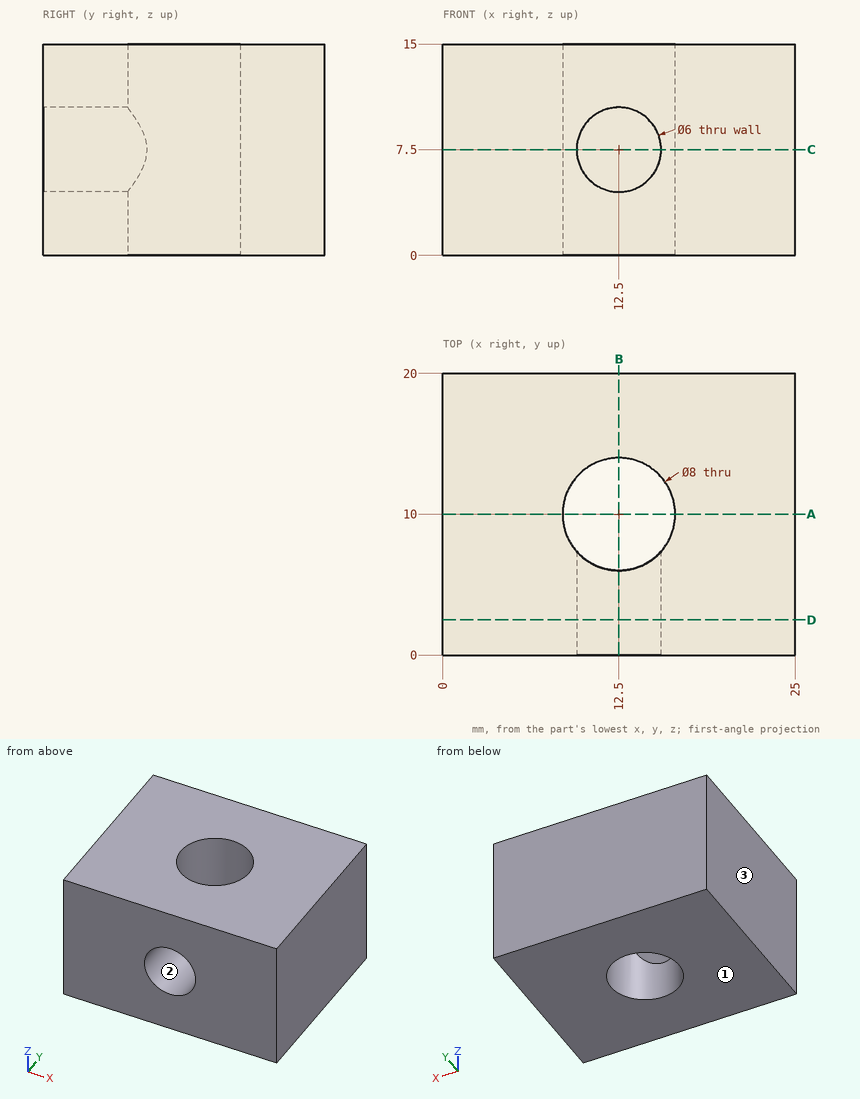
The drawing under review shows one solid part. Ordinate dimensions are in mm from its lowest x, y, z. Give positions to 0.01 mm unless a question says otherwise; leave off trailing zeros. Order: outer loops, then holes, each group sorted by start corner. A loop starts at its lowest first (then second) coordinate and runs counter-clockwise, first axis right, second up. Notation, with made-up numbers: (33, 25) -> (77, 25) arc R20 cw to (77, 38) -> close; hole circle Ø6 at (31.25, 68). An arc over 180 degrees is marked (long way). Write item = value, one per line.
1) We need section A-A, the plane y = 10. Give the boundary of the cut face in (x, z), and give its area (3 significant figures).
Findings:
outline = (0, 0) -> (8.5, 0) -> (8.5, 15) -> (0, 15) -> close; (16.5, 0) -> (25, 0) -> (25, 15) -> (16.5, 15) -> close
area = 255 mm^2
2) We need section D-D, the plane y = 2.5. Give the boundary of the cut face in (x, z), and give its area (3 significant figures).
Findings:
outline = (0, 0) -> (25, 0) -> (25, 15) -> (0, 15) -> close; hole circle Ø6 at (12.5, 7.5)
area = 347 mm^2
3) To check wall thickness, follow L1, parallel to Z at x = 12.5, y = 4; L2, parallel to X at y = 11.75, z = 6; L3, parallel to X at y = 8.75, z = 10.25. State the ranges of each line that lie inside material, in increasing order. Write a range as from..to.
Findings:
L1 = 0..4.5, 10.5..15
L2 = 0..8.9, 16.1..25
L3 = 0..8.7, 16.3..25
4) We need section C-C, the plane z = 7.5. Give the boundary of the cut face in (x, y), and give its area (3 significant figures).
Findings:
outline = (0, 0) -> (9.5, 0) -> (9.5, 7.35) arc R4 cw (long way) to (15.5, 7.35) -> (15.5, 0) -> (25, 0) -> (25, 20) -> (0, 20) -> close
area = 411 mm^2
5) Draft analysis for pull direction Z (two halves, no side actions). For the marked faces 1, 2 and 3, state which applies: pulls with the +Z half, pulls with the -Z half, needs draft (parallel to the pull), parting line crosses it, or undercut.
Findings:
face_1 = pulls with the -Z half
face_2 = undercut
face_3 = needs draft
6) Insertion check: pin 1 (3 mm diameter, centred on x = 11.5, y = 12, fed in from -Z). The pin has a flat end and moves straight along its axis. Give the tip position at first contact, or say it passes through.
Findings:
pin_1 = through
7) We need section B-B, the plane x = 12.5. Give the boundary of the cut face in (y, z).
Findings:
outline = (0, 0) -> (6, 0) -> (6, 4.5) -> (0, 4.5) -> close; (0, 10.5) -> (6, 10.5) -> (6, 15) -> (0, 15) -> close; (14, 0) -> (20, 0) -> (20, 15) -> (14, 15) -> close
